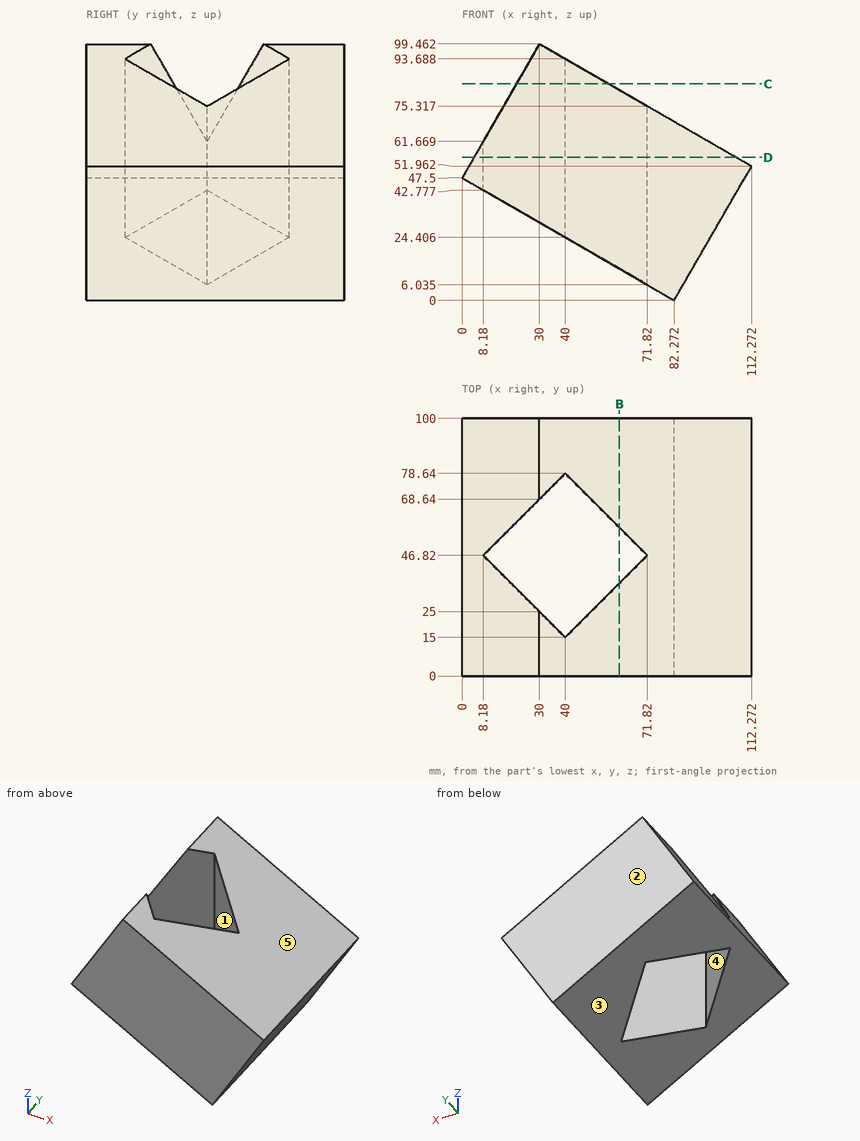
Geometry: see drawing. Coordinates: mm, zero at the bounding-box minimum. A direction names the side the tool comes from. Coordinates: 2 decimals unless noted, no trailing zeros. Order: outer loops, then holes, each group sorted by start corner. A loop starts at its lowest first (then second) coordinate and runs counter-clockwise, first axis right, second up. Notation, with made-up numbers: (-5.5, 12) -> (9.5, 12) arc R32 ccw to (9.5, 45) -> close; hole circle Ø9 at (-7, 54.25). An arc over 180 degrees is marked (long way). Write each question's results on one line, items separated by ' | '. Start each with the question number.
1) Mould query, pull axis X, two halves, no side actions, for the marked faces 1, 2 and 3. Classes: released by +X, released by -X, zero draft, split by the parting line, or undercut.
2) First-contact query: pin 1 (10 mm diameter, centred on x = 54.5, y = 74.5, fed in from -Z); pin 2 (2 mm diameter, centred on y = 23, z = 55.5, fed in from +X) (1 decimal); pin 3 (6 mm diameter, centred on y = 79.5, z = 16, fed in from -X) (1 decimal). Flat tips, straight axial feed; report the tip coordinate or a pass-through.
3) Cut plane D-D, the plane z = 55.5. Output: boundary loops of the cut face in (x, y), and give its area (3 significant figures).
4) Set-up query: the marked faces 4 and 5. Return all of +Z, -Z, +X, -X, +Y, -Y with unobstructed straight access to the full face (end or side cutting, diameter ignored); none if empty.
5) Material intervals for line 1 along Y through (x, z) = (66, 72); line 2 along X through (y, z) = (31.5, 48) (1 decimal); line 3 along X through (y, z) = (62.5, 64.5) (1 decimal), sorted ascending.
6) Cut plane B-B, the plane x = 61. Output: boundary loops of the cut face in (y, z).
7) Cut plane C-C, the plane z = 84. Output: boundary loops of the cut face in (x, y), and give its area (3 significant figures).
Checks:
1) face 1: undercut | face 2: zero draft | face 3: released by -X
2) pin 1: z = 13.15 | pin 2: x = 107.9 | pin 3: x = 49.4
3) outline: (4.62, 0) -> (106.14, 0) -> (106.14, 100) -> (4.62, 100) -> close; hole (8.18, 46.82) -> (40, 15) -> (71.82, 46.82) -> (40, 78.64) -> close | area: 8,130 mm^2
4) face 4: +Z, -Z | face 5: +Z, +X, +Y, -Y
5) line 1: 0 to 41, 52.64 to 100 | line 2: 0.3 to 23.5, 56.5 to 110 | line 3: 9.8 to 23.9, 56.1 to 90.6
6) outline: (0, 12.28) -> (36, 12.28) -> (36, 81.56) -> (0, 81.56) -> close; (57.64, 12.28) -> (100, 12.28) -> (100, 81.56) -> (57.64, 81.56) -> close
7) outline: (21.07, 0) -> (56.78, 0) -> (56.78, 31.78) -> (40, 15) -> (21.07, 33.93) -> close; (21.07, 59.71) -> (40, 78.64) -> (56.78, 61.86) -> (56.78, 100) -> (21.07, 100) -> close | area: 1,940 mm^2
